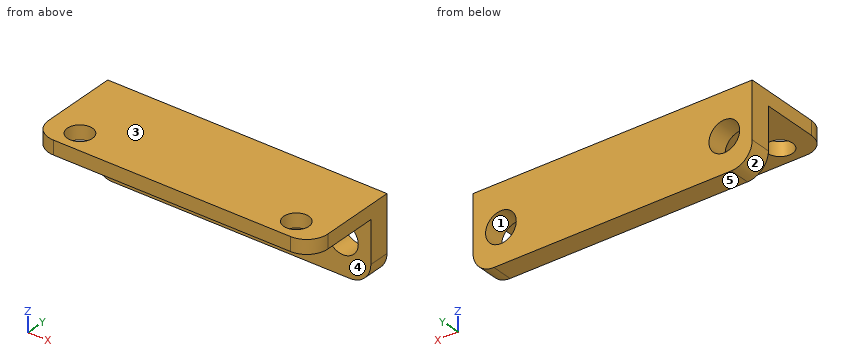
```python
from build123d import *

# Parameters (mm, degrees)
CYLINDER001_R            = 2.2
CYLINDER001_DEPTH        = 10
ARRAY005_Y_COUNT         = 2
ARRAY005_Y_PITCH         = 32
CYLINDER008_R            = 1.8
CYLINDER008_DEPTH        = 10
ARRAY004_Y_COUNT         = 2
ARRAY004_Y_PITCH         = 31
ARRAY004_PLACEMENT_ANGLE = 90
BOX007_W                 = 2
BOX007_H                 = 40
BOX007_DEPTH             = 11
FILLET004_R              = 3
BOX006_W                 = 11
BOX006_H                 = 40
BOX006_DEPTH             = 3
FILLET003_R              = 3
CUT005_PITCH_ANGLE       = 90
CUT005_PLACEMENT_ANGLE   = -90


with BuildPart() as pcb_hole_array:
    # Cylinder001 → Cylinder001 (new body)
    with BuildSketch(Plane.XY):
        Circle(CYLINDER001_R)
    extrude(amount=CYLINDER001_DEPTH)

    # Array005 Y: pcb hole array ×2


with BuildPart() as pcb_hole_array_1:
    add(pcb_hole_array.part)
    with Locations(*[(0, i * ARRAY005_Y_PITCH, 0) for i in range(1, ARRAY005_Y_COUNT)]):
        add(pcb_hole_array.part)


with BuildPart() as pcb_hole_array_2:
    # Array005 placement: moved
    add(pcb_hole_array_1.part.moved(Location((6, 4, -3))))


with BuildPart() as fusion010:
    # Cylinder008 → Cylinder008 (new body)
    with BuildSketch(Plane.XY):
        Circle(CYLINDER008_R)
    extrude(amount=CYLINDER008_DEPTH)

    # Array004 Y: Fusion010 ×2


with BuildPart() as fusion010_1:
    add(fusion010.part)
    with Locations(*[(0, i * ARRAY004_Y_PITCH, 0) for i in range(1, ARRAY004_Y_COUNT)]):
        add(fusion010.part)


with BuildPart() as fusion010_2:
    # Array004 placement: moved
    add(fusion010_1.part.moved(Location((0, 4.5, 8))).rotate(Axis((0, 4.5, 8), (0, 1, 0)), ARRAY004_PLACEMENT_ANGLE))

    # Fusion010: union pcb hole array
    add(pcb_hole_array_2.part)


with BuildPart() as fillet004:
    # Box007 → Box007 (new body)
    with BuildSketch(Plane.XY):
        with Locations((1, 20)):
            Rectangle(BOX007_W, BOX007_H)
    extrude(amount=BOX007_DEPTH)

    # Fillet004
    fillet004_edges = [fillet004.edges().sort_by_distance(p)[0] for p in [
        (1, 0, 11),
        (1, 40, 11),
    ]]
    fillet(fillet004_edges, radius=FILLET004_R)


with BuildPart() as pcb_holder_cut:
    # Box006 → Box006 (new body)
    with BuildSketch(Plane.XY.offset(-3)):
        with Locations((5.5, 20)):
            Rectangle(BOX006_W, BOX006_H)
    extrude(amount=BOX006_DEPTH)

    # Fillet003
    fillet003_edges = [pcb_holder_cut.edges().sort_by_distance(p)[0] for p in [
        (11, 0, -1.5),
        (11, 40, -1.5),
    ]]
    fillet(fillet003_edges, radius=FILLET003_R)

    # Fusion011: union Fillet004
    add(fillet004.part)

    # Cut005: cut Fusion010
    add(fusion010_2.part, mode=Mode.SUBTRACT)


with BuildPart() as pcb_holder_cut_1:
    # Cut005 pitch: moved
    add(pcb_holder_cut.part.rotate(Axis((0, 0, 0), (0, 1, 0)), CUT005_PITCH_ANGLE))


with BuildPart() as pcb_holder_cut_2:
    # Cut005 placement: moved
    add(pcb_holder_cut_1.part.moved(Location((-32.3, 68, 64.6))).rotate(Axis((-32.3, 68, 64.6), (0, 0, 1)), CUT005_PLACEMENT_ANGLE))


solid = pcb_holder_cut_2.part
```
The listing builds one solid part. Answer for the finished solid, in the listing's coordinates (mm). Face numbers are marked on the shaded views. A direction names the side the tool comes from. Round coordinates to 2 decimals unless told otherwise and drop trailing zeros. Write each loop counter-clockwise with the first axis right and the second up, starting at its lowest first coordinate (ties: lowest second). Pieces come first, ordered by that corner, then holes. Notation, with made-up numbers: (78, 64.25) -> (123, 64.25) arc R18 cw to (123, 83.25) -> close; hole circle Ø4 at (-39, -26). An arc over 180 degrees is marked (long way). Answer as a JSON object with one key per item and string values. Group by question number.
Q1. Straight lines are drawn through the part: line 1 along X through (y, z) = (69.55, 58.6); line 2 along X through (y, z) = (69, 59.25); line 3 along Z through (x, y) = (-28, 65.5). For each, find the intervals that lie inside material, in ascending order.
Q2. Section D-D (y = 70.25) is taken. Write down the section's boundary in (x, z).
Q3. Section C-C (x = -28.3) is taken. Write down the section's boundary in (y, z).
Q4. Section A-A (z = 63.5) is taken. Write down the section's boundary in (x, y).
Q5. Section B-B (z = 58.6) is taken. Write down the section's boundary in (x, y), plus the area to 3 significant figures.
Q6. Which of the six approach directions +Z, -Z, +X, -X, +Y, -Y give full straight-line access (tool end or side, diameter ignored) to the marked faces 4 and 5?
Q7. Determine the mould class of the marked faces 1, 2 and 3 for opening direction Z: pulls with the +Z half, pulls with the -Z half, needs draft (parallel to the pull), parting line crosses it, or undercut.
Q8. Each of these flat-tipped pins is pushed along its axis until it touches: pin 1 Ø3 at (x, y) = (-4.5, 59.5) entering from -Z; pin 2 Ø2.5 at (x, z) = (-6.5, 59) entering from -Y. Where does it stop, or does it pass through?
Check values:
{
 "1": {"line 1": "-32.3 to -30.5, -26.1 to 1.5, 5.9 to 7.7", "line 2": "-32.3 to -30.4, -26.2 to 1.6, 5.8 to 7.7", "line 3": "62.6 to 64.6"},
 "2": {"outline": "(-32.3, 56.6) arc R3 ccw to (-29.3, 53.6) -> (4.7, 53.6) arc R3 ccw to (7.7, 56.6) -> (7.7, 64.6) -> (-32.3, 64.6) -> close; hole circle Ø4.4 at (-28.3, 58.6); hole circle Ø4.4 at (3.7, 58.6)"},
 "3": {"outline": "(57, 62.6) -> (58.27, 62.6) -> (58.27, 64.6) -> (57, 64.6) -> close; (61.73, 62.6) -> (68, 62.6) -> (68, 60.8) -> (71, 60.8) -> (71, 64.6) -> (61.73, 64.6) -> close; (68, 53.6) -> (71, 53.6) -> (71, 56.4) -> (68, 56.4) -> close"},
 "4": {"outline": "(-32.3, 60) arc R3 ccw to (-29.3, 57) -> (4.7, 57) arc R3 ccw to (7.7, 60) -> (7.7, 71) -> (-32.3, 71) -> close; hole circle Ø3.6 at (-27.8, 60); hole circle Ø3.6 at (3.2, 60)"},
 "5": {"outline": "(-32.3, 68) -> (-30.5, 68) -> (-30.5, 71) -> (-32.3, 71) -> close; (-26.1, 68) -> (1.5, 68) -> (1.5, 71) -> (-26.1, 71) -> close; (5.9, 68) -> (7.7, 68) -> (7.7, 71) -> (5.9, 71) -> close", "area": "93.6 mm^2"},
 "6": {"face 4": "-Z, +X, -X, -Y", "face 5": "-Z, +X, -X, +Y, -Y"},
 "7": {"face 1": "undercut", "face 2": "pulls with the -Z half", "face 3": "pulls with the +Z half"},
 "8": {"pin 1": "z = 62.6", "pin 2": "y = 68"}
}
